from build123d import *

# Parameters (mm, degrees)
F0_R      = 2
F1_DEPTH  = 10
F2_R      = 5
F4_R      = 2
F5_DEPTH  = 10
F7_R      = 5
F7_2_R    = 5
F8_R      = 2
F8_2_R    = 2
F10_DEPTH = 25
F11_R     = 1.5
F12_R     = 1.75
F13_DEPTH = 12.5
F15_W     = 9
F15_H     = 20
F16_DEPTH = 10
F17_W     = 6
F17_H     = 20
F18_DEPTH = 25
F21_R     = 2
F22_DEPTH = 30
F24_R     = 2
F25_DEPTH = 12.5
F27_R     = 2
F28_R     = 2
F29_DEPTH = 8
F30_R     = 2
F31_R     = 2
F32_R     = 1.75
F33_DEPTH = 25
F32_R_2   = 2
F37_ANGLE = 90
F40_W     = 60
F40_H     = 10
F40_R     = 2
F41_DEPTH = 8
F43_R     = 1.5


with BuildPart() as f1:
    # F0 (on Top) → F1 (new body)
    with BuildSketch(Plane.XY):
        Polygon((0, 70), (0, 75), (-20, 75), (-30, 75), (-50, -75), (-40, -75), (0, -75), (0, -65), (-38.6666666667, -65), (-30.8, -6), (0, -6), (0, 0), (0, 6), (-29.2, 6), (-21.3333333333, 65), (0, 65), align=None)
        with Locations((-15, 0)):
            Circle(F0_R, mode=Mode.SUBTRACT)
        with Locations((-10.4101235047, 70)):
            Circle(F0_R, mode=Mode.SUBTRACT)
    extrude(amount=F1_DEPTH)

    # F2
    f2_edges = [f1.edges().sort_by_distance(p)[0] for p in [
        (-21.333333, 65, 5),
        (-30.8, -6, 5),
        (-29.2, 6, 5),
        (-38.666667, -65, 5),
        (-50, -75, 5),
    ]]
    fillet(f2_edges, radius=F2_R)

    # F3: F1 across plane


with BuildPart() as f1_1:
    add(f1.part)
    add(f1.part.mirror(Plane.YZ))

    # F4 (on Top) → F5 (join)
    with BuildSketch(Plane.XY):
        with BuildLine():
            Line((0, 80), (0, 75))
            Line((0, 75), (10, 75))
            Line((10, 75), (30, 75))
            Line((30, 75), (13.3333333333, 200))
            Line((13.3333333333, 200), (4.5, 200))
            Line((4.5, 200), (4.5, 192))
            ThreePointArc((4.5, 192), (3.1819805153, 188.8180194847), (0, 187.5))
            Line((0, 187.5), (0, 170.1721444783))
            Line((0, 170.1721444783), (7.3103807362, 170.1721444783))
            Line((7.3103807362, 170.1721444783), (10, 150))
            Line((10, 150), (18.6666666667, 85))
            Line((18.6666666667, 85), (10, 85))
            Line((10, 85), (0, 85))
            Line((0, 85), (0, 80))
        make_face()
        with Locations((10, 80)):
            Circle(F4_R, mode=Mode.SUBTRACT)
    extrude(amount=F5_DEPTH)


with BuildPart() as f6_1:
    # F6: instance of F1
    add(f1_1.part.mirror(Plane.YZ))

    # F7
    f7_edges = [f6_1.edges().sort_by_distance(p)[0] for p in [
        (-7.310381, 170.172144, 5),
        (-18.666667, 85, 5),
        (-13.333333, 200, 5),
    ]]
    fillet(f7_edges, radius=F7_R)

    # F8#2
    f8_2_edges = [f6_1.edges().sort_by_distance(p)[0] for p in [
        (-4.5, 200, 5),
    ]]
    fillet(f8_2_edges, radius=F8_2_R)


with BuildPart() as f1_2:
    add(f1_1.part)

    # F7#2
    f7_2_edges = [f1_2.edges().sort_by_distance(p)[0] for p in [
        (7.310381, 170.172144, 5),
        (18.666667, 85, 5),
        (13.333333, 200, 5),
    ]]
    fillet(f7_2_edges, radius=F7_2_R)

    # F8
    f8_edges = [f1_2.edges().sort_by_distance(p)[0] for p in [
        (4.5, 200, 5),
    ]]
    fillet(f8_edges, radius=F8_R)

    add(f6_1.part)  # F10 merges F6_1
    # F9 (on Top) → F10 (join)
    with BuildSketch(Plane.XY):
        Polygon((0, -6), (0, 0), (0, 6), (-6, 6), (-6, -6), align=None)
    extrude(amount=F10_DEPTH)

    # F11
    f11_edges = [f1_2.edges().sort_by_distance(p)[0] for p in [
        (-6, -6, 17.5),
        (-6, 0, 25),
        (-3, -6, 25),
        (-6, 6, 17.5),
        (-3, 6, 25),
    ]]
    fillet(f11_edges, radius=F11_R)


with BuildPart() as f13:
    # F12 (on Right) → F13 (new body, symmetric)
    with BuildSketch(Plane.YZ):
        with Locations((0, 20)):
            Circle(F12_R)
    extrude(amount=F13_DEPTH, both=True)


with BuildPart() as f13b:
    # F12 (on Right) → F13, piece 2 (new body, symmetric)
    with BuildSketch(Plane.YZ):
        with Locations((0, 15)):
            Circle(F12_R)
    extrude(amount=F13_DEPTH, both=True)


with BuildPart() as f1_3:
    add(f1_2.part)

    # F14: cut F13b, F13
    add(f13b.part, mode=Mode.SUBTRACT)
    add(f13.part, mode=Mode.SUBTRACT)


with BuildPart() as f16:
    # F15 (on Top) → F16 (new body)
    with BuildSketch(Plane.XY):
        Polygon((0, 65), (15, 65), (15, 85), (0, 85), (0, 75), align=None)
        Polygon((-6, 65), (0, 65), (0, 75), (0, 85), (-6, 85), align=None)
        with Locations((-10.5, 75)):
            Rectangle(F15_W, F15_H)
    extrude(amount=F16_DEPTH)


with BuildPart() as f18:
    # F17 (on Top) → F18 (new body)
    with BuildSketch(Plane.XY):
        with Locations((-3, 75)):
            Rectangle(F17_W, F17_H)
    extrude(amount=F18_DEPTH)


with BuildPart() as f16_1:
    add(f16.part)

    # F19: union F18
    add(f18.part)


with BuildPart() as f16_2:
    # F20: moved
    add(f16_1.part.moved(Location((0, 0, 10))))


with BuildPart() as f22:
    # F21 (on Top) → F22 (new body)
    with BuildSketch(Plane.XY):
        with Locations((-10, 80)):
            Circle(F21_R)
    extrude(amount=F22_DEPTH)


with BuildPart() as f22b:
    # F21 (on Top) → F22, piece 2 (new body)
    with BuildSketch(Plane.XY):
        with Locations((10, 80)):
            Circle(F21_R)
    extrude(amount=F22_DEPTH)


with BuildPart() as f22c:
    # F21 (on Top) → F22, piece 3 (new body)
    with BuildSketch(Plane.XY):
        with Locations((-10.4, 70)):
            Circle(F21_R)
    extrude(amount=F22_DEPTH)


with BuildPart() as f22d:
    # F21 (on Top) → F22, piece 4 (new body)
    with BuildSketch(Plane.XY):
        with Locations((10.4, 70)):
            Circle(F21_R)
    extrude(amount=F22_DEPTH)


with BuildPart() as f16_3:
    add(f16_2.part)

    # F23: cut F22d, F22c, F22b, F22
    add(f22d.part, mode=Mode.SUBTRACT)
    add(f22c.part, mode=Mode.SUBTRACT)
    add(f22b.part, mode=Mode.SUBTRACT)
    add(f22.part, mode=Mode.SUBTRACT)


with BuildPart() as f25:
    # F24 (on Right) → F25 (new body, symmetric)
    with BuildSketch(Plane.YZ):
        with Locations((80, 27.2266920656)):
            Circle(F24_R)
    extrude(amount=F25_DEPTH, both=True)


with BuildPart() as f25b:
    # F24 (on Right) → F25, piece 2 (new body, symmetric)
    with BuildSketch(Plane.YZ):
        with Locations((70, 27.2266920656)):
            Circle(F24_R)
    extrude(amount=F25_DEPTH, both=True)


with BuildPart() as f16_4:
    add(f16_3.part)

    # F26: cut F25b, F25
    add(f25b.part, mode=Mode.SUBTRACT)
    add(f25.part, mode=Mode.SUBTRACT)

    # F27
    f27_edges = [f16_4.edges().sort_by_distance(p)[0] for p in [
        (-6, 65, 27.5),
        (-3, 65, 35),
        (-10.5, 65, 20),
        (-15, 65, 15),
        (7.5, 65, 20),
        (15, 65, 15),
        (15, 75, 10),
        (-15, 75, 10),
        (-6, 75, 35),
        (-10.5, 85, 20),
        (-15, 85, 15),
        (-6, 85, 27.5),
        (-3, 85, 35),
        (7.5, 85, 20),
        (15, 85, 15),
    ]]
    fillet(f27_edges, radius=F27_R)


with BuildPart() as f29:
    # F28 (on Right) → F29 (new body)
    with BuildSketch(Plane.YZ):
        Polygon((-6, 10), (0, 10), (6, 10), (6, 25), (65, 35), (65, 20), (75, 20), (85, 20), (85, 35), (85, 120), (75, 120), (-6, 25), align=None)
        Polygon((17.4430621123, 37.0821219176), (23.9249371816, 44.6843210729), (75, 104.5871725266), (75, 45), (64.1585427985, 45), (51.9163602293, 42.9250538018), align=None, mode=Mode.SUBTRACT)
        with Locations((80, 95)):
            Circle(F28_R, mode=Mode.SUBTRACT)
        with Locations((80, 110)):
            Circle(F28_R, mode=Mode.SUBTRACT)
    extrude(amount=F29_DEPTH)

    # F30
    f30_edges = [f29.edges().sort_by_distance(p)[0] for p in [
        (4, 75, 104.587173),
        (4, 75, 45),
        (4, 17.443062, 37.082122),
        (4, 65, 35),
        (4, 6, 25),
        (4, -6, 25),
    ]]
    fillet(f30_edges, radius=F30_R)

    # F31
    f31_edges = [f29.edges().sort_by_distance(p)[0] for p in [
        (8, 46.246648, 70.864105),
        (8, 34.73905, 72.780367),
        (8, 35.165784, 29.943353),
        (8, 85, 70),
    ]]
    fillet(f31_edges, radius=F31_R)


with BuildPart() as f33:
    # F32 (on Right) → F33 (new body)
    with BuildSketch(Plane.YZ):
        with Locations((0, 20)):
            Circle(F32_R)
    extrude(amount=F33_DEPTH)


with BuildPart() as f33b:
    # F32 (on Right) → F33, piece 2 (new body)
    with BuildSketch(Plane.YZ):
        with Locations((0, 15)):
            Circle(F32_R)
    extrude(amount=F33_DEPTH)


with BuildPart() as f33c:
    # F32 (on Right) → F33, piece 3 (new body)
    with BuildSketch(Plane.YZ):
        with Locations((70, 27.25)):
            Circle(F32_R_2)
    extrude(amount=F33_DEPTH)


with BuildPart() as f33d:
    # F32 (on Right) → F33, piece 4 (new body)
    with BuildSketch(Plane.YZ):
        with Locations((80, 27.25)):
            Circle(F32_R_2)
    extrude(amount=F33_DEPTH)


with BuildPart() as f29_1:
    add(f29.part)

    # F34: cut F33d, F33c, F33b, F33
    add(f33d.part, mode=Mode.SUBTRACT)
    add(f33c.part, mode=Mode.SUBTRACT)
    add(f33b.part, mode=Mode.SUBTRACT)
    add(f33.part, mode=Mode.SUBTRACT)


with BuildPart() as f29_2:
    # F37: moved
    add(f29_1.part.rotate(Axis((0, -39.3833108246, 0), (0, -1, 0)), F37_ANGLE))


with BuildPart() as f29_3:
    # F38: moved
    add(f29_2.part.moved(Location((120, -60, 0))))


with BuildPart() as f39_1:
    # F39: instance of F29
    add(f29_3.part.mirror(Plane.YZ))


with BuildPart() as f41:
    # F40 (on Top) → F41 (new body)
    with BuildSketch(Plane.XY):
        with Locations((0, 20)):
            Rectangle(F40_W, F40_H)
        with Locations((-25, 20)):
            Circle(F40_R, mode=Mode.SUBTRACT)
        with Locations((-10, 20)):
            Circle(F40_R, mode=Mode.SUBTRACT)
        with Locations((10, 20)):
            Circle(F40_R, mode=Mode.SUBTRACT)
        with Locations((25, 20)):
            Circle(F40_R, mode=Mode.SUBTRACT)
    extrude(amount=F41_DEPTH)


with BuildPart() as f41_1:
    # F42: moved
    add(f41.part.moved(Location((0, 0, 8))))

    # F43
    f43_edges = [f41_1.edges().sort_by_distance(p)[0] for p in [
        (0, 15, 16),
        (30, 15, 12),
        (30, 25, 12),
        (30, 20, 16),
        (-30, 20, 16),
        (-30, 15, 12),
        (-30, 25, 12),
        (0, 25, 16),
    ]]
    fillet(f43_edges, radius=F43_R)


solid = f41_1.part
The model under review builds one solid part; all positions refer to its coordinate system, in mm. Give positions to 0.01 mm unless a question says otherwise; leave off trailing zeros. Order: outer loops, then holes, each group sorted by start corner. A loop starts at its lowest first (then second) coordinate and runs counter-clockwise, first axis right, second up. Notation, with made-up numbers: M 38.5,23.25 L 56.5,23.25 A16 ccw 56.5,54.25 Z; hole C -16,16 d4. An arc over 180 degrees is marked long. Use one line per item in the form item = value. Start each with the question number.
Item 1: We need section A-A on x = 10. Give the boundary of the cut face in (y, z), plus the area to 3 significant figures.
Item 2: We need section C-C on y = 20. Give the boundary of the cut face in (x, z), plus the area to 3 significant figures.
Item 3: We need section B-B on z = 10.25. Give the boundary of the cut face in (x, y), plus the area to 3 significant figures.
Item 4: The part is to be moulded in two halves that separate along Y. For faces 1 (the cylindrical face through (10, 22, 12)), 2 (the flat face through (0, 25, 11)), 3 (the cylindrical face through (29.57, 20.05, 15.55)), say which applies: pulls with the +Y half, pulls with the -Y half, needs draft (parallel to the pull), parting line crosses it, or undercut.
Item 5: To check wall thickness, follow line 1 along Y through (x, z) = (-25, 11.5); line 2 along X through (y, z) = (18.5, 14.75); line 3 along X through (y, z) = (20.5, 13). State the ranges of each line that lie inside material, in increasing order. Write a range as from..to.
Item 6: We need section D-D on x = 26. Give the boundary of the cut face in (y, z).
Completed:
q1.outline = M 15,8 L 18,8 L 18,16 L 16.5,16 A1.5 ccw 15,14.5 Z; M 22,8 L 25,8 L 25,14.5 A1.5 ccw 23.5,16 L 22,16 Z
q1.area = 47.0 mm²
q2.outline = M -30,8 L -27,8 L -27,16 L -28.5,16 A1.5 ccw -30,14.5 Z; M -23,8 L -12,8 L -12,16 L -23,16 Z; M -8,8 L 8,8 L 8,16 L -8,16 Z; M 12,8 L 23,8 L 23,16 L 12,16 Z; M 27,8 L 30,8 L 30,14.5 A1.5 ccw 28.5,16 L 27,16 Z
q2.area = 351 mm²
q3.outline = M -30,16.5 A1.5 ccw -28.5,15 L 28.5,15 A1.5 ccw 30,16.5 L 30,23.5 A1.5 ccw 28.5,25 L -28.5,25 A1.5 ccw -30,23.5 Z; hole C -25,20 d4; hole C -10,20 d4; hole C 10,20 d4; hole C 25,20 d4
q3.area = 548 mm²
q4.face_1 = undercut
q4.face_2 = pulls with the +Y half
q4.face_3 = needs draft
q5.line_1 = 15..18, 22..25
q5.line_2 = -29.98..-26.32, -23.68..-11.32, -8.68..8.68, 11.32..23.68, 26.32..29.98
q5.line_3 = -30..-26.94, -23.06..-11.94, -8.06..8.06, 11.94..23.06, 26.94..30
q6.outline = M 15,8 L 18.27,8 L 18.27,16 L 16.5,16 A1.5 ccw 15,14.5 Z; M 21.73,8 L 25,8 L 25,14.5 A1.5 ccw 23.5,16 L 21.73,16 Z
